Can you work these out from the drawing? Everything is in mm from the part's minimum corner. A direction names the side the tool comes from. Round coordinates to 2 decimals unless told otherwise and drop trailing zeros. Loops run counter-clockwise (first coordinate to the right, second up) from the corner with the lowest first, then second, coordinate; pieces in that order, holes last. Notation, with made-up numbers: M 88,22 L 100,22 A7 ccw 100,31 Z; hole C 40,43.5 d7. An arc over 180 degrees is marked long. Answer in a Markdown table with one row per item.
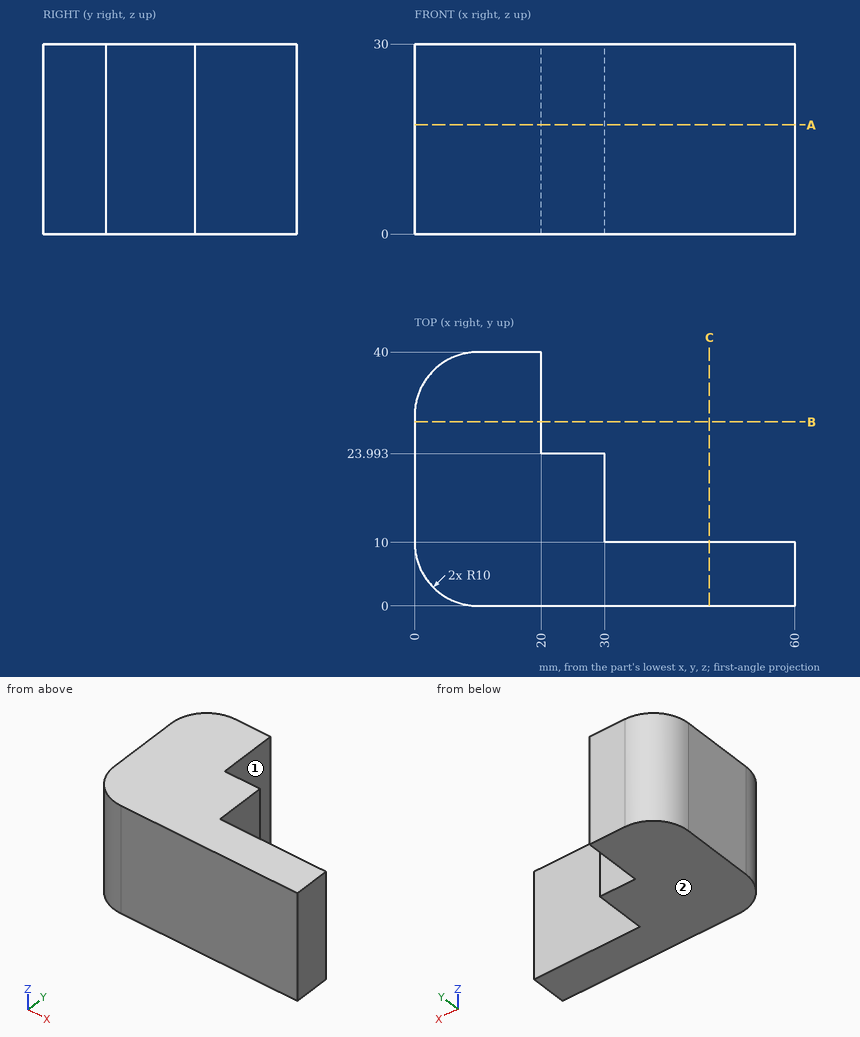
1) Will these pins go through, and if not, where does the flat tip stop? P1, Ø4, axis at y = 19.5, z = 15.5, coming from the +X side; P2, Ø15, axis at x = 45, z = 17, coming from the +Y side; P3, Ø8, axis at y = 30.5, z = 21.5, coming from the +X side.
Computed:
| item | result |
|---|---|
| P1 | stops at x = 30 |
| P2 | stops at y = 10 |
| P3 | stops at x = 20 |
2) I want a section at C-C, the plane x = 46.5. Please give me the cut outline in (y, z).
Computed:
| item | result |
|---|---|
| outline | M 0,0 L 10,0 L 10,30 L 0,30 Z |
3) I want a section at B-B, the plane y = 29. Please give me the cut outline in (x, z), plus the area to 3 significant figures.
Computed:
| item | result |
|---|---|
| outline | M 0,0 L 20,0 L 20,30 L 0,30 Z |
| area | 600 mm² |
4) I want a section at A-A, the plane z = 17.25. Please give me the cut outline in (x, y), plus the area to 3 significant figures.
Computed:
| item | result |
|---|---|
| outline | M 0,10 A10 ccw 10,0 L 60,0 L 60,10 L 30,10 L 30,23.99 L 20,23.99 L 20,40 L 10,40 A10 ccw 0,30 Z |
| area | 1,300 mm² |
5) I need wall thicknesses on line 1 (Y direction, x = 40.5, z = 1.75); line 2 (X direction, y = 24.5, z = 9.25); line 3 (X direction, y = 20.5, z = 16.5). Which ranges of each line are inside material? Lowest first, please.
Computed:
| item | result |
|---|---|
| line 1 | y = 0 to 10 |
| line 2 | x = 0 to 20 |
| line 3 | x = 0 to 30 |
6) Which directions (+Z, -Z, +X, -X, +Y, -Y) give clear straight access to the entire face, cutting with the end or side of a thin tool? Please do the marked faces 1 and 2.
Computed:
| item | result |
|---|---|
| face 1 | +Z, -Z, +X, +Y |
| face 2 | -Z, +X, -X, +Y, -Y |
